Verification items for the finished model (mm, model axes). Face numbers are marked on the shaded views. Coordinates: 2 decimals unless noted, no trailing zeros. Loops run counter-clockwise (first coordinate to the right, second up) from the corner with the lowest first, then second, coordinate; pieces in that order, holes last. Notation, with made-up numbers: (2.5, 72.5) - (6.5, 72.5) arc R15 cw to (6.5, 88.5) - close; hole circle Ø8 at (41.5, 22.25). An arc over 180 degrees is marked (long way). Answer as CSV lines item,"result". Start each with the question number.
1. Release check for a two-part mould opening along X. For the marked faces 1 and 2 record: pulls with the +X half, pulls with the -X half, needs draft (parallel to the pull), parting line crosses it, or undercut.
2. Cross-section at C-C (x = 10). Enter the section's corners in (y, z).
3. Material ranges on line 1 (Z direction, x = 93, y = 1.7); line 2 (X direction, y = 1.55, z = -94); line 3 (Z direction, x = 35, y = 1) (3 decimals), recorded low to high. Write a range as [from, to].
4. Gauge pin test, flat ends, axial feed: P1, Ø10, axis at x = 17, z = -23.5, coming from the -Y side; P2, Ø5, axis at x = 66, z = -13, coming from the +Y side. Record the tip position at first contact, or that the pin passes through.
5. Cross-section at A-A (z = -29.5). Enter the section's corners in (x, y) (3 decimals), plus the area to 3 significant figures.
6. Cross-section at D-D (z = -99). Enter the section's corners in (x, y), plus the area to 3 significant figures.
7. Cross-section at B-B (y = 3.2). Enter the section's corners in (x, z), plus the area to 3 significant figures.
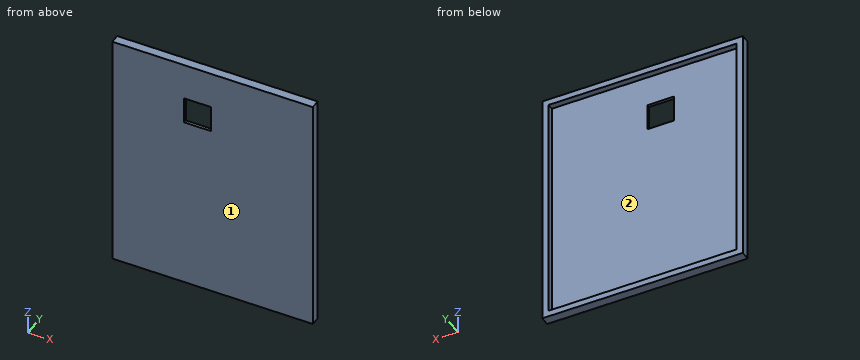
Autodesk Inventor part; units mm, degrees
ref_plane "YZ Plane" through (0, 0, 0) normal (1, 0, 0) x (0, 1, 0)
ref_plane "XZ Plane" through (0, 0, 0) normal (0, 1, 0) x (-1, 0, 0)
ref_plane "XY Plane" through (0, 0, 0) normal (0, 0, 1) x (1, 0, 0)
sketch "Esboço1" plane through (0, 0, 0) normal (0, 1, 0) x (-1, 0, 0)
  line L0 (0, 0) -> (-97.4, 0)
  line L1 (-97.4, 0) -> (-97.4, -117.4)
  line L2 (-97.4, -117.4) -> (0, -117.4)
  line L3 (0, -117.4) -> (0, 0)
  line L4 (-3, -3) -> (-94.4, -3)
  line L5 (-94.4, -3) -> (-94.4, -114.4)
  line L6 (-94.4, -114.4) -> (-3, -114.4)
  line L7 (-3, -114.4) -> (-3, -3)
  point P0 (-48.7, -114.4)
  point P1 (-48.7, 0)
  point P2 (-48.7, -3)
  dimension "d2" = 3
  dimension "d3" = 3
  dimension "d4" = 3
  dimension "d5" = 3
  dimension "d6" = 91.4
  dimension "d7" = 111.4
extrude "Extrusão1" add sketch "Esboço1" along normal blind 1.5 contours L7 L6 L5 L4
extrude "Extrusão2" add sketch "Esboço1" along normal blind 4.5
sketch "Esboço2" plane through (0, 0, 0) normal (0, -1, 0) x (1, 0, 0)
  line L0 (47.925, -30.975) -> (34.925, -30.975)
  line L1 (34.925, -30.975) -> (34.925, -17.975)
  line L2 (34.925, -17.975) -> (47.925, -17.975)
  line L3 (47.925, -17.975) -> (47.925, -30.975)
  line L4 (0, 0) -> (97.4, 0)
  line L5 (0, -117.4) -> (0, 0)
  dimension "d12" = 13
  dimension "d13" = 13
  dimension "d16" = 17.975
  dimension "d17" = 34.925
extrude "Extrusão3" cut sketch "Esboço2" against normal blind 10
properties part number "Tampa_3DPrint"
Values follow:
1,face 1,"needs draft"
1,face 2,"undercut"
2,outline,"(0, -117.4) - (4.5, -117.4) - (4.5, -114.4) - (1.5, -114.4) - (1.5, -3) - (4.5, -3) - (4.5, 0) - (0, 0) - close"
3,line 1,"z = [-117.4, -114.4], [-3, 0]"
3,line 2,"x = [0, 3], [94.4, 97.4]"
3,line 3,"z = [-117.4, -30.975], [-17.975, 0]"
4,P1,"stops at y = 0"
4,P2,"stops at y = 1.5"
5,outline,"(0, 0) - (34.925, 0) - (34.925, 1.5) - (3, 1.5) - (3, 4.5) - (0, 4.5) - close; (47.925, 0) - (97.4, 0) - (97.4, 4.5) - (94.4, 4.5) - (94.4, 1.5) - (47.925, 1.5) - close"
5,area,"145 mm²"
6,outline,"(0, 0) - (97.4, 0) - (97.4, 4.5) - (94.4, 4.5) - (94.4, 1.5) - (3, 1.5) - (3, 4.5) - (0, 4.5) - close"
6,area,"164 mm²"
7,outline,"(0, -117.4) - (97.4, -117.4) - (97.4, 0) - (0, 0) - close; hole (3, -114.4) - (94.4, -114.4) - (94.4, -3) - (3, -3) - close"
7,area,"1,250 mm²"
